Autodesk Inventor part; units mm, degrees
ref_plane "YZ Plane" through (0, 0, 0) normal (1, 0, 0) x (0, 1, 0)
ref_plane "XZ Plane" through (0, 0, 0) normal (0, 1, 0) x (-1, 0, 0)
ref_plane "XY Plane" through (0, 0, 0) normal (0, 0, 1) x (1, 0, 0)
sketch "Szkic1" plane through (0, 0, 0) normal (0, 0, 1) x (1, 0, 0)
  line L0 (-50, 50) -> (50, 50)
  line L1 (50, 50) -> (50, -50)
  line L2 (50, -50) -> (-50, -50)
  line L3 (-50, -50) -> (-50, 50)
  point P0 (0, 0)
  point P1 (0, 50)
  point P2 (-50, 0)
  dimension "d0" = 100
  dimension "d1" = 100
extrude "Wyciągnięcie proste1" add sketch "Szkic1" along normal blind 10
sketch "Szkic2" plane through (0, 0, 10) normal (0, 0, 1) x (1, 0, 0)
  line L0 (-50, -50) -> (50, -50)
  line L1 (50, -50) -> (50, 50)
  line L2 (-50, -50) -> (50, -50)
  line L3 (50, -50) -> (50, -25)
  line L4 (50, -25) -> (-50, -25)
  line L5 (-50, -25) -> (-50, -50)
  point P0 (0, 0)
  dimension "d4" = 25
extrude "Wyciągnięcie proste2" add sketch "Szkic2" along normal blind 100
sketch "Szkic3" plane through (-50, -25, 10) normal (0, 1, 0) x (1, 0, 0)
  circle A0 centre (49.7287, -50.229) radius 50
  circle A1 centre (36.7287, -37.229) radius 2.75
  circle A2 centre (36.7287, -63.229) radius 2.75
  circle A3 centre (62.7287, -37.229) radius 2.75
  circle A4 centre (62.7287, -63.229) radius 2.75
  circle A5 centre (78.013, -78.5133) radius 2.75
  circle A6 centre (89.7287, -50.229) radius 2.75
  circle A7 centre (78.013, -21.9447) radius 2.75
  circle A8 centre (49.7287, -10.229) radius 2.75
  circle A9 centre (21.4444, -21.9447) radius 2.75
  circle A10 centre (9.7287, -50.229) radius 2.75
  circle A11 centre (21.4444, -78.5133) radius 2.75
  circle A12 centre (49.7287, -90.229) radius 2.75
  point P0 (50, 10)
extrude "Wyciągnięcie proste3" cut sketch "Szkic3" against normal blind 100 contours A1 | A2 | A3 | A4 | A5 | A6 | A7 | A8 | A9 | A10 | A11 | A12
properties part number "uchwyt chwytak"
Part model, mm, in its own coordinate system. A direction names the side the tool comes from. Coordinates: 2 decimals unless noted, no trailing zeros. Loops run counter-clockwise (first coordinate to the right, second up) from the corner with the lowest first, then second, coordinate; pieces in that order, holes last. Notation, with made-up numbers: (-34.5, 80) - (-0.5, 80) arc R24 ccw to (-0.5, 113) - close; hole circle Ø11 at (9, 47.25). An arc over 180 degrees is marked (long way). Write each question's results on one line, items separated by ' | '. Start each with the question number.
Q1. Slice it at D-D on z = 78.5. Give the cut face in (x, y), and give its area (3 significant figures).
Q2. Slice it at A-A on x = -41. Give the cut face in (y, z).
Q3. Probe line 1 along X through (y, z) = (-39.5, 89.5); line 2 along X through (y, z) = (-29.5, 100.5); line 3 along Z through (x, y) = (-12, -30.5). List the from-to ranges inside material, lowest first.
Q4. Drop flat-ended pins along their axis: pin 1 Ø9 at (x, z) = (-40.27, 60.23) entering from +Y; pin 2 Ø1 at (x, y) = (-29, 27) entering from +Z. Give the stop position or say it passes through.
Q5. Slice it at C-C on y = 28. Give the cut face in (x, z).
Q6. Which spindle directions (+Z, -Z, +X, -X, +Y, -Y) get a long thin tool onto all of the face, cutting with end or side? Do faces 4 (the cylindrical face through (-27.287, -37.325, 90.953)), 5 (the flat face through (1, -25, 59)). Say none if no direction does.
Q7. Slice it at B-B on x = -7. Give the cut face in (y, z).
Q8. Two-plate mould, pull along Z, no slides. Class faces 1 (the flat face through (50, -26, 47)), 2 (the flat face through (-1, -37, 110)), 3 (the cylindrical face through (12.4, -37.3, 70.5)): +Z half, -Z half, draft (parallel to the pull), parting line (faces both ways), or undercut.
Answer:
1) outline: (-50, -50) - (50, -50) - (50, -25) - (-50, -25) - close | area: 2,500 mm2
2) outline: (-50, 0) - (50, 0) - (50, 10) - (-25, 10) - (-25, 57.58) - (-50, 57.58) - close; (-50, 62.88) - (-25, 62.88) - (-25, 110) - (-50, 110) - close
3) line 1: x = -50 to -31.12, -25.99 to 25.45, 30.58 to 50 | line 2: x = -50 to -3.01, 2.47 to 50 | line 3: z = 0 to 44.79, 49.67 to 70.79, 75.67 to 110
4) pin 1: stops at y = -25 | pin 2: stops at z = 10
5) outline: (-50, 0) - (50, 0) - (50, 10) - (-50, 10) - close
6) face 4: +Y, -Y | face 5: +Z, +X, -X, +Y
7) outline: (-50, 0) - (50, 0) - (50, 10) - (-25, 10) - (-25, 110) - (-50, 110) - close
8) face 1: draft | face 2: +Z half | face 3: undercut
